Geometry: final body of the model. Coordinates: model frame, mm. Give positions to 0.01 mm unless a question says otherwise; leave off trailing zeros. Order: outer loops, then holes, each group sorted by start corner. A loop starts at its lowest first (then second) coordinate and runs counter-clockwise, first axis right, second up. Notation, with made-up numbers: (-13.5, -0.5) - (9.5, -0.5) arc R25 cw to (9.5, 24.5) - close; hole circle Ø10 at (45, 17). An arc over 180 degrees is marked (long way). One line per item, written item: value.
```python
from build123d import *

# Parameters (mm, degrees)
SKETCH1_R           = 124.46
SKETCH1_R_2         = 85.8139
BOSS_EXTRUDE1_DEPTH = 1.5875
SKETCH2_R           = 3.302
CUT_EXTRUDE1_DEPTH  = 1.5875
CIRPATTERN1_COUNT   = 12
CUT_EXTRUDE2_DEPTH  = 1.5875
CIRPATTERN2_COUNT   = 12


with BuildPart() as part:
    # Sketch1 → Boss-Extrude1 (new body)
    with BuildSketch(Plane(origin=(0, 0, 0), x_dir=(1, 0, 0), z_dir=(0, 1, 0))):
        Circle(SKETCH1_R)
        Circle(SKETCH1_R_2, mode=Mode.SUBTRACT)
    extrude(amount=BOSS_EXTRUDE1_DEPTH)

    # Sketch2 → Cut-Extrude1 (cut)
    with BuildSketch(Plane(origin=(0, 1.5875, 0), x_dir=(1, 0, 0), z_dir=(0, 1, 0))):
        with Locations((0, 111.76)):
            Circle(SKETCH2_R)
    cut_extrude1 = extrude(amount=-CUT_EXTRUDE1_DEPTH, mode=Mode.SUBTRACT)

    # CirPattern1: Cut-Extrude1 ×12 about axis
    cirpattern1_axis = Axis((0, 0, 0), (0, 1, 0))
    for i in range(1, CIRPATTERN1_COUNT):
        add(cut_extrude1.rotate(cirpattern1_axis, i * 360 / CIRPATTERN1_COUNT), mode=Mode.SUBTRACT)

    # Sketch4 → Cut-Extrude2 (cut)
    with BuildSketch(Plane(origin=(0, 1.5875, 0), x_dir=(1, 0, 0), z_dir=(0, 1, 0))):
        with BuildLine():
            Line((0, 124.46), (0, 155.146488396))
            Line((0, 155.146488396), (77.573244198, 134.360800259))
            Line((77.573244198, 134.360800259), (62.23, 107.785521755))
            ThreePointArc((62.23, 107.785521755), (54.190877213, 109.374169747), (46.855001911, 105.722289245))
            ThreePointArc((46.855001911, 105.722289245), (26.879703963, 100.316420883), (12.283522673, 114.985689189))
            ThreePointArc((12.283522673, 114.985689189), (7.756408554, 121.816248125), (0, 124.46))
        make_face()
    cut_extrude2 = extrude(amount=-CUT_EXTRUDE2_DEPTH, mode=Mode.SUBTRACT)

    # CirPattern2: Cut-Extrude2 ×12 about axis
    cirpattern2_axis = Axis((0, 0, 0), (0, 1, 0))
    for i in range(1, CIRPATTERN2_COUNT):
        add(cut_extrude2.rotate(cirpattern2_axis, i * 360 / CIRPATTERN2_COUNT), mode=Mode.SUBTRACT)


solid = part.part
```
1) Mould query, pull axis Z, two halves, no side actions, for faces 1 (the face through (-27.17, 0.8, 100.24)), 2 (the face through (73.653, 0.805, -73.224)), 3 (the face through (-74, 0, -47)). Classes: released by +Z, released by -Z, zero draft, split by the parting line, or undercut.
Answers below:
face 1: released by +Z
face 2: undercut
face 3: zero draft
2) Material intervals for line 1 along X through (y, z) = (0.7, -55.88) (3 decimals); line 2 along Z through (x, y) = (-58.5, 0.4), sorted ascending.
Answers below:
line 1: -109.487 to -100.089, -93.485 to -65.126, 65.126 to 93.485, 100.089 to 109.487
line 2: -109.21 to -98.8, -94.78 to -62.78, 62.78 to 94.78, 98.8 to 109.21
3) Section C-C, the plane z = 55.88. Return loops of the section in (x, y) (1 decimal), then the cut area to 3 significant figures.
Answers below:
outline: (-109.5, 0) - (-100.1, 0) - (-100.1, 1.6) - (-109.5, 1.6) - close; (-93.5, 0) - (-65.1, 0) - (-65.1, 1.6) - (-93.5, 1.6) - close; (65.1, 0) - (93.5, 0) - (93.5, 1.6) - (65.1, 1.6) - close; (100.1, 0) - (109.5, 0) - (109.5, 1.6) - (100.1, 1.6) - close
area: 120 mm^2
4) Section D-D, the plane y = 1.3. Count the separate pieces of the cut face and the enclosed holes in it, then the cut area to 3 significant figures.
Answers below:
separate pieces: 1
enclosed holes: 13
area: 16,800 mm^2
5) Section B-B, the plane x = 55.88. Return loops of the section in (y, z) (1 decimal).
Answers below:
outline: (0, -109.5) - (1.6, -109.5) - (1.6, -100.1) - (0, -100.1) - close; (0, -93.5) - (1.6, -93.5) - (1.6, -65.1) - (0, -65.1) - close; (0, 65.1) - (1.6, 65.1) - (1.6, 93.5) - (0, 93.5) - close; (0, 100.1) - (1.6, 100.1) - (1.6, 109.5) - (0, 109.5) - close
6) Section A-A, the plane z = 27. Return loops of the section in (x, y), then the cut area to 3 significant figures.
Answers below:
outline: (-100.28, 0) - (-81.46, 0) - (-81.46, 1.59) - (-100.28, 1.59) - close; (81.46, 0) - (100.28, 0) - (100.28, 1.59) - (81.46, 1.59) - close
area: 59.8 mm^2
7) First-contact query: pin 1 (5.5 mm diameter, centred on x = -111.76, z = 0, fed in from -Y). Flat tip, straight axial feed; report the tip coordinate or a pass-through.
Answers below:
pin 1: through
